Here's how the part is built. I have some questions about the finished solid (model axes, mm). A direction names the side the tool comes from. Round coordinates to 2 decimals unless told otherwise and drop trailing zeros. Loops run counter-clockwise (first coordinate to the right, second up) from the corner with the lowest first, then second, coordinate; pieces in that order, holes last. Notation, with made-up numbers: (53.25, 15.5) - (72.25, 15.5) arc R26 cw to (72.25, 38.5) - close; hole circle Ø2 at (59, 81). An arc over 180 degrees is marked (long way). Answer as a JSON object with one key per item and string values. Group by question number.
1) I want a section at A-A, the plane z = -13. Please give me the cut outline in (x, y).
2) I want a section at B-B, the plane x = 2.75. Give the number of separate pieces and of enclosed holes in the cut face, then the cut area to 3 significant figures.
3) I want a section at C-C, the plane y = -90.5. Please give me the cut outline in (x, z).
4) If I drill on line 1 along Y through (x, z) = (1.25, -51); line 2 along Y through (x, z) = (6, -39.5); line 3 along Y through (x, z) = (6.5, -2.5), over which ranges is the centre line in solid material (lowest first)? Write a range as [from, to].
5) If we mould it in two halves opening along Y, with no side actions, what happens to faces 1 (the face through (9, -9, 1)), 2 (the face through (4.44, -172.7, 3.06)), 3 (the face through (4.437, 151.806, 40.582))? For each: pulls with the +Y half, pulls with the -Y half, needs draft (parallel to the pull), parting line crosses it, or undercut.
6) Which directions (+Z, -Z, +X, -X, +Y, -Y) give clear straight access to the entire face, cutting with the end or side of a thin tool? Please do faces 4 (the face through (4.44, 172.34, 40.98)), 5 (the face through (4.44, 172.16, -41.29)), 6 (the face through (6.146, -162.241, 36.376)).
7) I want a section at D-D, the plane z = 18.5. Please give me the cut outline in (x, y), then the cut area to 3 significant figures.
8) Will these pins go through, and if not, where does the flat tip stop? P1, Ø7.5, axis at y = -158.88, z = -37.12, coming from the +X side; P2, Ø4.5, axis at x = 6.5, y = 43.5, coming from the -Z side; P3, Ø2.5, axis at x = 3.5, y = -19, coming from the +Z side; P4, Ø6, axis at y = -233.12, z = -37.12, coming from the -X side.
from build123d import *

# Parameters (mm, degrees)
SKETCH1_R                                           = 23.5
BOSS_EXTRUDE1_DEPTH                                 = 9
CSK_FOR_M6_COUNTERSUNK_FLAT_HEAD_SCREW1_D           = 6.6
CSK_FOR_M6_COUNTERSUNK_FLAT_HEAD_SCREW1_CSINK_D     = 12.6
CSK_FOR_M6_COUNTERSUNK_FLAT_HEAD_SCREW1_CSINK_ANGLE = 90


with BuildPart() as part:
    # Sketch1 → Boss-Extrude1 (new body)
    with BuildSketch(Plane(origin=(0, 0, 0), x_dir=(0, 0, -1), z_dir=(1, 0, 0))):
        with BuildLine():
            Line((-30.310889132, 178.5), (-51.961524227, 166))
            ThreePointArc((-51.961524227, 166), (-40.390167668, 151.630704809), (-25, 141.456439427))
            Line((-25, 141.456439427), (-25, -141.456439427))
            ThreePointArc((-25, -141.456439427), (0, -256), (25, -141.456439427))
            Line((25, -141.456439427), (25, 141.456439427))
            ThreePointArc((25, 141.456439427), (40.390167668, 151.630704809), (51.961524227, 166))
            Line((51.961524227, 166), (30.310889132, 178.5))
            ThreePointArc((30.310889132, 178.5), (0, 231), (-30.310889132, 178.5))
        make_face()
        with Locations((0, -196)):
            Circle(SKETCH1_R, mode=Mode.SUBTRACT)
    extrude(amount=BOSS_EXTRUDE1_DEPTH)

    # CSK for M6 Countersunk Flat Head Screw1 (through all)
    with Locations(Plane(origin=(9, 0, 0), x_dir=(0, 0, -1), z_dir=(1, 0, 0))):
        with Locations((-37.123106012, -158.876893988), (0, -143.5), (37.123106012, -158.876893988), (52.5, -196), (37.123106012, -233.123106012), (0, -248.5), (-37.123106012, -233.123106012), (-52.5, -196)):
            CounterSinkHole(CSK_FOR_M6_COUNTERSUNK_FLAT_HEAD_SCREW1_D / 2, CSK_FOR_M6_COUNTERSUNK_FLAT_HEAD_SCREW1_CSINK_D / 2, counter_sink_angle=CSK_FOR_M6_COUNTERSUNK_FLAT_HEAD_SCREW1_CSINK_ANGLE)


solid = part.part
Outcome:
{
 "1": {"outline": "(0, -254.57) - (9, -254.57) - (9, -215.58) - (0, -215.58) - close; (0, -176.42) - (9, -176.42) - (9, 228.5) - (0, 228.5) - close"},
 "2": {"separate pieces": "1", "enclosed holes": "9", "area": "29,400 mm^2"},
 "3": {"outline": "(0, -25) - (9, -25) - (9, 25) - (0, 25) - close"},
 "4": {"line 1": "[-227.61, -198.94], [-193.06, -164.39], [164.39, 166.56]", "line 2": "[-241.16, -235.41], [-230.83, -161.17], [-156.59, -150.84], [150.84, 173.19]", "line 3": "[-255.95, -251.36], [-245.64, -219.37], [-172.63, -146.36], [-140.64, 230.91]"},
 "5": {"face 1": "needs draft", "face 2": "undercut", "face 3": "undercut"},
 "6": {"face 4": "+Z, +X, -X", "face 5": "-Z, +X, -X", "face 6": "+X"},
 "7": {"outline": "(0, -253.08) - (9, -253.08) - (9, -210.49) - (0, -210.49) - close; (0, -181.51) - (9, -181.51) - (9, 225.71) - (0, 225.71) - close", "area": "4,050 mm^2"},
 "8": {"P1": "x = 6.45", "P2": "z = -25", "P3": "z = 25", "P4": "through"}
}
